Can you work these out from the model? Positions are in its coordinate system, mm. A direction names the side the tool comes from. Give positions to 0.01 mm unless a question says otherwise; leave off trailing zeros. Order: outer loops, then holes, each group sorted by start corner. A loop starts at its lowest first (then second) coordinate and runs counter-clockwise, first axis right, second up.
Item 1: I want a section at B-B, the plane y = 31.5. Write out the boundary of the cut face in (x, z), then the cut area to 3 significant figures.
Item 2: Which directions (+Z, -Z, +X, -X, +Y, -Y) give clear straight access to the entire face, cutting with the end or side of a thin tool? Please do faces 4 (the flat face through (7.5, 2, 0)), 5 (the flat face through (0, 44, 0)), 6 (the cylindrical face through (9.3, 29.85, 2.93)).
Item 3: If I drill on line 1 along Z through (x, y) = (20, 1.8); line 2 along X through (y, z) = (2.3, 20); line 3 along X through (y, z) = (2.5, 6), over which ranges is the centre line in solid material (lowest first)?
Item 4: I'm going to push flat-ended pins straight in: pin 1 Ø10 at (y, z) = (34, 18) entering from -X; pin 2 Ø8 at (x, y) = (0, 31.5) entering from +Z; pin 3 Ø4 at (x, z) = (-20, 20) entering from +Y; pin 4 Ø2 at (y, z) = (11, 8) entering from +X. Where does each tip first touch, or does it pass through?
Item 5: I want a section at D-D, the plane y = 39.5. Write out the boundary of the cut face in (x, z).
Item 6: I want a section at A-A, the plane x = 0. Write out the boundary of the cut face in (y, z).
Item 7: I want a section at C-C, the plane z = 20. Count the separate pieces of the cut face and the enclosed holes in it, then the cut area to 3 significant figures.
Item 8: If we mould it in two halves opening along Z, with no side actions, what happens to faces 1 (the flat face through (11, 4, 20)), 2 (the cylindrical face through (-23.4, 2.03, -23.43)), 3 (the cylindrical face through (18.99, 1.97, 18.89))? For each: +Z half, -Z half, draft (parallel to the pull), parting line (faces both ways), or undercut.
Autodesk Inventor part; units mm, degrees
ref_plane "YZ Plane" through (0, 0, 0) normal (1, 0, 0) x (0, 1, 0)
ref_plane "XZ Plane" through (0, 0, 0) normal (0, 1, 0) x (-1, 0, 0)
ref_plane "XY Plane" through (0, 0, 0) normal (0, 0, 1) x (1, 0, 0)
sketch "Sketch1" plane through (0, 0, 0) normal (0, 1, 0) x (-1, 0, 0)
  line L0 (24, 24) -> (-24, 24)
  line L1 (-24, 24) -> (-24, -24)
  line L2 (-24, -24) -> (24, -24)
  line L3 (24, -24) -> (24, 24)
  line L4 (24, 24) -> (-24, -24) construction
  line L5 (-24, 24) -> (24, -24) construction
  point P0 (0, 0)
  dimension "d0" = 48
  dimension "d1" = 48
extrude "Extrusion1" add sketch "Sketch1" along normal blind 4
sketch "Sketch2" plane through (0, 4, 0) normal (0, 1, 0) x (1, 0, 0)
  circle A0 centre (0, 0) radius 15
  dimension "d4" = 30
extrude "Extrusion2" add sketch "Sketch2" along normal blind 15
fillet "Fillet1" radius 7 1 edges at (-15, 4, 0)
sketch "Sketch4" plane through (0, 4, 0) normal (0, 1, 0) x (1, 0, 0)
  line L0 (20, 20) -> (-20, 20) construction
  line L1 (-20, 20) -> (-20, -20) construction
  line L2 (-20, -20) -> (20, -20) construction
  line L3 (20, -20) -> (20, 20) construction
  line L4 (20, 20) -> (-20, -20) construction
  line L5 (-20, 20) -> (20, -20) construction
  point P0 (0, 0)
  dimension "d11" = 40
  dimension "d12" = 40
hole "Hole1" at (-20, 4, 20) at (-20, 4, -20) at (20, 4, 20) at (20, 4, -20) direction (0, -1, 0) diameter 3 end through all
fillet "Fillet2" radius 2 4 edges at (24, 2, 24) (-24, 2, 24) (24, 2, -24) (-24, 2, -24)
sketch "Sketch5" plane through (22, 0, -24) normal (0, 0, -1) x (-1, 0, 0)
  line L0 (14.5, -3) -> (29.5, -3)
  line L1 (29.5, -3) -> (29.5, 3)
  line L2 (29.5, 3) -> (14.5, 3)
  line L3 (14.5, 3) -> (14.5, -3)
  line L4 (14.5, -3) -> (29.5, 3) construction
  line L5 (29.5, -3) -> (14.5, 3) construction
  point P0 (22, 0)
  dimension "d21" = 15
  dimension "d22" = 6
extrude "Extrusion4" cut sketch "Sketch5" against normal blind 80
sketch "Sketch6" plane through (0, 19, 0) normal (0, 1, 0) x (1, 0, 0)
  circle A0 centre (0, 0) radius 9.75
  dimension "d25" = 19.5
extrude "Extrusion5" add sketch "Sketch6" along normal blind 25
fillet "Fillet3" radius 3 1 edges at (-9.75, 44, 0)
sketch "Sketch7" plane through (-22, 4, 24) normal (0, 0, 1) x (1, 0, 0)
  line L0 (22, -4) -> (22, 27.5) construction
  dimension "d29" = 31.5
hole "Hole2" at (0, 31.5, 24) direction (0, 0, -1) diameter 6 end through all
properties part number "adaptor"
Results list:
1. outline: (-3, -9.28) - (-3, 9.28) arc R9.75 ccw to start; (3, -9.28) arc R9.75 ccw to (3, 9.28) - close
1. area: 184 mm2
2. face 4: +Z, -Z, -Y
2. face 5: +Z, -Z, +X, -X, +Y
2. face 6: +Y
3. line 1: z = -24 to -21.5, -18.5 to 18.5, 21.5 to 24
3. line 2: x = -24 to -21.5, -18.5 to -7.5, 7.5 to 18.5, 21.5 to 24
3. line 3: x = -24 to -7.5, 7.5 to 24
4. pin 1: passes through
4. pin 2: stops at z = 9.75
4. pin 3: stops at y = 4
4. pin 4: stops at x = 13.27
5. outline: circle Ø19.5 at (0, 0)
6. outline: (3, -24) - (4, -24) - (4, -22) arc R7 cw to (11, -15) - (19, -15) - (19, -9.75) - (28.5, -9.75) - (28.5, 9.75) - (19, 9.75) - (19, 15) - (11, 15) arc R7 cw to (4, 22) - (4, 24) - (3, 24) - close; (34.5, -9.75) - (41, -9.75) arc R3 ccw to (44, -6.75) - (44, 6.75) arc R3 ccw to (41, 9.75) - (34.5, 9.75) - close
7. separate pieces: 3
7. enclosed holes: 0
7. area: 126 mm2
8. face 1: draft
8. face 2: -Z half
8. face 3: undercut
